from build123d import *

# Parameters (mm, degrees)
BOX_W        = 2.4
BOX_H        = 24
BOX_DEPTH    = 22
BOX001_W     = 2.4
BOX001_H     = 24
BOX001_DEPTH = 22
BOX002_W     = 2.4
BOX002_H     = 24
BOX002_DEPTH = 22
BOX003_W     = 2.4
BOX003_H     = 24
BOX003_DEPTH = 22
BOX004_W     = 33
BOX004_H     = 30
BOX004_DEPTH = 22


with BuildPart() as ranura1:
    # Box → Box (new body)
    with BuildSketch(Plane.XY):
        with Locations((1.2, 12)):
            Rectangle(BOX_W, BOX_H)
    extrude(amount=BOX_DEPTH)


with BuildPart() as ranura002:
    # Box001 → Box001 (new body)
    with BuildSketch(Plane(origin=(8, 0, 0), x_dir=(1, 0, 0), z_dir=(0, 0, 1))):
        with Locations((1.2, 12)):
            Rectangle(BOX001_W, BOX001_H)
    extrude(amount=BOX001_DEPTH)


with BuildPart() as ranura003:
    # Box002 → Box002 (new body)
    with BuildSketch(Plane(origin=(16, 0, 0), x_dir=(1, 0, 0), z_dir=(0, 0, 1))):
        with Locations((1.2, 12)):
            Rectangle(BOX002_W, BOX002_H)
    extrude(amount=BOX002_DEPTH)


with BuildPart() as fusion:
    # Box003 → Box003 (new body)
    with BuildSketch(Plane(origin=(24, 0, 0), x_dir=(1, 0, 0), z_dir=(0, 0, 1))):
        with Locations((1.2, 12)):
            Rectangle(BOX003_W, BOX003_H)
    extrude(amount=BOX003_DEPTH)

    # Fusion: union Ranura1, Ranura002, Ranura003
    add(ranura1.part)
    add(ranura002.part)
    add(ranura003.part)


with BuildPart() as fusion_1:
    # Fusion placement: moved
    add(fusion.part.moved(Location((3, 3, 1))))


with BuildPart() as cut:
    # Box004 → Box004 (new body)
    with BuildSketch(Plane.XY):
        with Locations((16.5, 15)):
            Rectangle(BOX004_W, BOX004_H)
    extrude(amount=BOX004_DEPTH)

    # Cut: cut Fusion
    add(fusion_1.part, mode=Mode.SUBTRACT)


solid = cut.part
Geometry check sheet. Reference: the model listing, model coordinates, mm. A direction names the side the tool comes from. Give positions to 0.01 mm unless a question says otherwise; leave off trailing zeros. Order: outer loops, then holes, each group sorted by start corner. A loop starts at its lowest first (then second) coordinate and runs counter-clockwise, first axis right, second up. Notation, with made-up numbers: M -28,42 L 13,42 A20 cw 13,56 Z; hole C -21,37.25 d5. An arc over 180 degrees is marked long. Use a Markdown table: item, result.
Item 1: Material ranges on line 1 along X through (y, z) = (18.5, 12); line 2 along Y through (x, z) = (20.5, 4.75); line 3 along Z through (x, y) = (11.5, 23), recorded low to high.
Answers follow:
| item | result |
|---|---|
| line 1 | x = 0 to 3, 5.4 to 11, 13.4 to 19, 21.4 to 27, 29.4 to 33 |
| line 2 | y = 0 to 3, 27 to 30 |
| line 3 | z = 0 to 1 |
Item 2: Depth check by flat-ended pin: P1, Ø1.2, axis at x = 20, y = 14.5, coming from the +Z side. Enter the tip coordinate at first touch or a pass-through.
Answers follow:
| item | result |
|---|---|
| P1 | stops at z = 1 |
Item 3: Tool access check on faces 1 (the flat face through (4, 15, 1)), 2 (the flat face through (16, 0, 11)). Record the directions out of +Z, -Z, +X, -X, +Y, -Y that give a thin tool (end or side, any length) a straight path to the whole face; none if there is none.
Answers follow:
| item | result |
|---|---|
| face 1 | +Z |
| face 2 | +Z, -Z, +X, -X, -Y |
Item 4: Draft check along X on faces 3 (the flat face through (0, 15, 11)), 4 (the flat face through (16, 15, 22)), 5 (the flat face through (5.4, 15, 11)), 6 (the flat face through (28, 3, 11)). Enter one of: +X half, -X half, draft (parallel to the pull), parting line (faces both ways), or undercut.
Answers follow:
| item | result |
|---|---|
| face 3 | -X half |
| face 4 | draft |
| face 5 | undercut |
| face 6 | undercut |
Item 5: Section check A-A (z = 9.75). Record the cut outline in (x, y), and give its area (3 significant figures).
Answers follow:
| item | result |
|---|---|
| outline | M 0,0 L 33,0 L 33,30 L 0,30 Z; hole M 3,3 L 5.4,3 L 5.4,27 L 3,27 Z; hole M 11,3 L 13.4,3 L 13.4,27 L 11,27 Z; hole M 19,3 L 21.4,3 L 21.4,27 L 19,27 Z; hole M 27,3 L 29.4,3 L 29.4,27 L 27,27 Z |
| area | 760 mm2 |
Item 6: Section check C-C (y = 10.5). Record the cut outline in (x, z), and give its area (3 significant figures).
Answers follow:
| item | result |
|---|---|
| outline | M 0,0 L 33,0 L 33,22 L 29.4,22 L 29.4,1 L 27,1 L 27,22 L 21.4,22 L 21.4,1 L 19,1 L 19,22 L 13.4,22 L 13.4,1 L 11,1 L 11,22 L 5.4,22 L 5.4,1 L 3,1 L 3,22 L 0,22 Z |
| area | 524 mm2 |
Item 7: Section check B-B (x = 4). Record the cut outline in (y, z), and give its area (3 significant figures).
Answers follow:
| item | result |
|---|---|
| outline | M 0,0 L 30,0 L 30,22 L 27,22 L 27,1 L 3,1 L 3,22 L 0,22 Z |
| area | 156 mm2 |
